The drawing under review shows one solid part. Ordinate dimensions are in mm from its lowest x, y, z. Give positions to 0.01 mm unless a question says otherwise; leave off trailing zeros. Loops run counter-clockwise (first coordinate to the right, second up) from the corner with the lowest first, then second, coordinate; pieces in that order, holes last. Notation, with made-up numbers: M 82,7 L 135,7 A19 ccw 135,13 Z; hole C 46.5,78.5 d10. An arc over 180 degrees is marked long. Write item = value, one per line. Start each with the question number.
1. Wall thickness on line 1 along X through (y, z) = (4.75, 41.5) (1 decimal); line 2 along X through (y, z) = (10.5, 12) (1 decimal); line 3 along Y through (x, z) = (13, 75) (1 decimal): over which ranges is each line inside the solid? List them lowest first. Write a range as from..to.
2. We need section B-B on x = 2.75. Give the boundary of the cut face in (y, z) (1 decimal).
3. We need section C-C on y = 5.5. Give the boundary of the cut face in (x, z) (1 decimal).
4. For pin 1 (4 mm diameter, centred on y = 7.5, z = 36.5, fed in from +X) (1 decimal); pin 2 (2 mm diameter, centred on y = 1.5, z = 63.5, fed in from -X), all flat-tipped, find the tip position at first contact; note any pin that passes through.
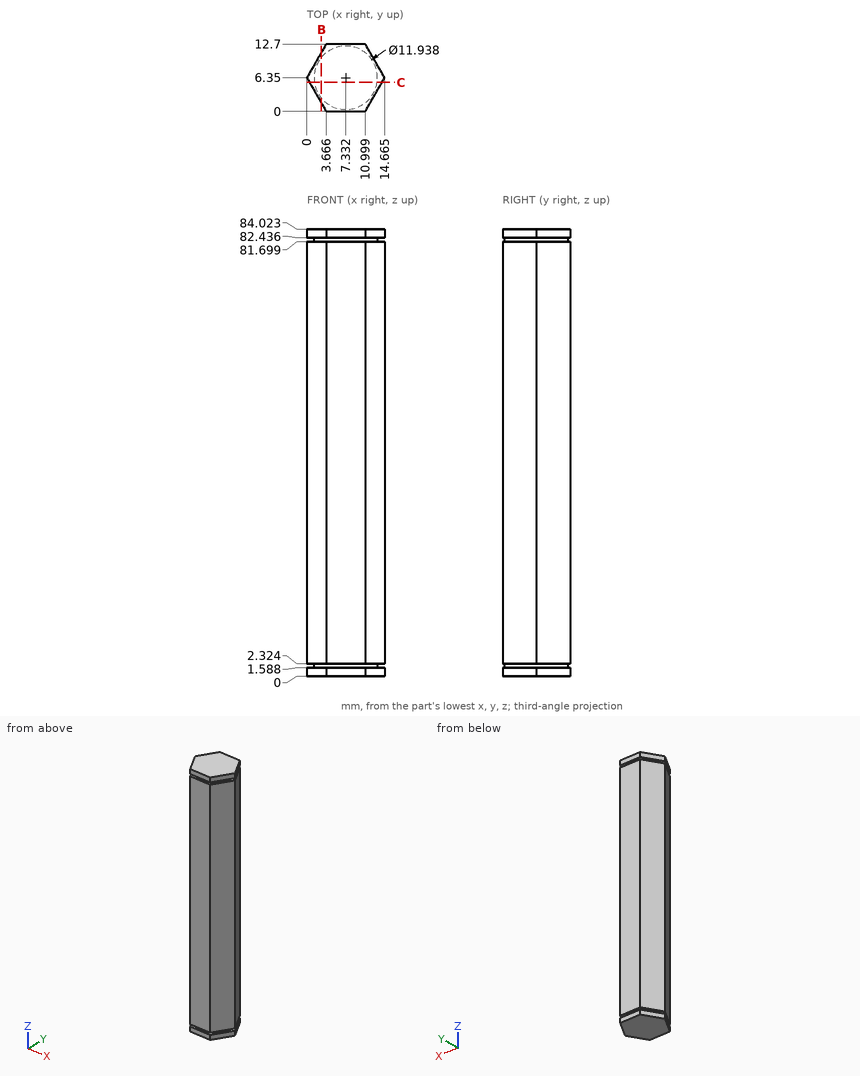
Final values:
q1.line_1 = 0.9..13.7
q1.line_2 = 2.4..12.3
q1.line_3 = 3.5..9.2
q2.outline = M 1.6,0 L 11.1,0 L 11.1,1.6 L 10.2,1.6 L 10.2,2.3 L 11.1,2.3 L 11.1,81.7 L 10.2,81.7 L 10.2,82.4 L 11.1,82.4 L 11.1,84 L 1.6,84 L 1.6,82.4 L 2.5,82.4 L 2.5,81.7 L 1.6,81.7 L 1.6,2.3 L 2.5,2.3 L 2.5,1.6 L 1.6,1.6 Z
q3.outline = M 0.5,0 L 14.2,0 L 14.2,1.6 L 13.2,1.6 L 13.2,2.3 L 14.2,2.3 L 14.2,81.7 L 13.2,81.7 L 13.2,82.4 L 14.2,82.4 L 14.2,84 L 0.5,84 L 0.5,82.4 L 1.4,82.4 L 1.4,81.7 L 0.5,81.7 L 0.5,2.3 L 1.4,2.3 L 1.4,1.6 L 0.5,1.6 Z
q4.pin_1 = 14.7
q4.pin_2 = 2.22
